Verification items for the finished model (mm, model axes). A direction names the side the tool comes from. Round coordinates to 2 decimals unless told otherwise and drop trailing zeros. Write each loop counter-clockwise with the first axis right and the second up, starting at its lowest first coordinate (ties: lowest second). Pieces come first, ordered by that corner, then holes. Notation, with made-up numbers: (6.5, 45.25) -> (65.5, 45.25) arc R21 cw to (65.5, 68.25) -> close; hole circle Ø1 at (41, 22.25). An arc over 180 degrees is marked (long way). Answer as a JSON object with one key per item and string values. Group by question number.
(1) Gauge pin test, flat ends, axial feed: pin 1 Ø16 at (x, y) = (-17, 7.5) entering from -Z; pin 2 Ø3 at (x, y) = (2.5, 34) entering from +Z; pin 3 Ø10 at (y, z) = (13, 18) entering from -X; pin 4 Ø3 at (x, z) = (4, 74) entering from -Y. Record the tip position at first contact, or that the pin passes through.
(2) Draft check along Z on faces 4 (the face through (-47, 10, -54)), 5 (the face through (-1, 80, -100)), 6 (the face through (-88.594, 80.14, 87.972)). Enter one of: released by +Z, released by -Z, zero draft, split by the parting line, or undercut.
(3) Sectioned sample at B-B on y = 77. Record the cut outline in (x, z), and give its area (3 significant figures).
(4) Scan lines: L1, parallel to X at y = 10.75, z = 50; L2, parallel to Y at x = 55, z = 47.5; L3, parallel to Y at x = -11, z = -85. Record each from-to range of solid material in increasing order. Write a range as from..to.
(5) Sectioned sample at A-A on x = 0. Record the cut outline in (y, z).
(6) Set-up check for faces 1 (the face through (-1, 20, -51)), 2 (the face through (-1, 10, -75)), 3 (the face through (68.986, 10.14, -69.297)): record each of +Z, -Z, +X, -X, +Y, -Y from which the full face is reachable in a straight line by a thin tool's end or side.
(7) Sectioned sample at D-D on z = 0. Record the cut outline in (x, y), and give its area (3 significant figures).
(8) Sectioned sample at C-C on z = -70. Record the cut outline in (x, y), and give its area (3 significant figures).
```python
from build123d import *

# Parameters (mm, degrees)
SKETCH_1_W      = 150
SKETCH_1_H      = 150
SKETCH_1_R      = 5
EXTRUDE_1_DEPTH = 20
FILLET_1_R      = 20
SKETCH_2_R      = 50
EXTRUDE_2_DEPTH = 50
SKETCH_3_W      = 200
SKETCH_3_H      = 200
EXTRUDE_3_DEPTH = 20
FILLET_2_R      = 40


with BuildPart() as part:
    # Эскиз1 → Бобышка-Вытянуть1 (new body)
    with BuildSketch(Plane(origin=(0, 0, 0), x_dir=(1, 0, 0), z_dir=(0, 1, 0))):
        Rectangle(SKETCH_1_W, SKETCH_1_H)
        with Locations(Location((-50, 50, 0), (0, 0, 270))):
            Circle(SKETCH_1_R, mode=Mode.SUBTRACT)
        with Locations(Location((50, 50, 0), (0, 0, 270))):
            Circle(SKETCH_1_R, mode=Mode.SUBTRACT)
        with Locations(Location((50, -50, 0), (0, 0, 270))):
            Circle(SKETCH_1_R, mode=Mode.SUBTRACT)
        with Locations(Location((-50, -50, 0), (0, 0, 270))):
            Circle(SKETCH_1_R, mode=Mode.SUBTRACT)
    extrude(amount=EXTRUDE_1_DEPTH)

    # Скругление1
    fillet_1_edges = [part.edges().sort_by_distance(p)[0] for p in [
        (-75, 10, 75),
        (-75, 10, -75),
        (75, 10, -75),
        (75, 10, 75),
    ]]
    fillet(fillet_1_edges, radius=FILLET_1_R)

    # Эскиз2 → Бобышка-Вытянуть2 (add)
    with BuildSketch(Plane(origin=(0, 20, 0), x_dir=(1, 0, 0), z_dir=(0, 1, 0))):
        with Locations(Location((0, 0, 0), (0, 0, 270))):
            Circle(SKETCH_2_R)
    extrude(amount=EXTRUDE_2_DEPTH)

    # Эскиз3 → Бобышка-Вытянуть3 (add)
    with BuildSketch(Plane(origin=(0, 70, 0), x_dir=(1, 0, 0), z_dir=(0, 1, 0))):
        Rectangle(SKETCH_3_W, SKETCH_3_H)
    extrude(amount=EXTRUDE_3_DEPTH)

    # Скругление2
    fillet_2_edges = [part.edges().sort_by_distance(p)[0] for p in [
        (100, 80, 100),
        (100, 80, -100),
        (-100, 80, -100),
        (-100, 80, 100),
    ]]
    fillet(fillet_2_edges, radius=FILLET_2_R)


solid = part.part
```
Computed values:
{
 "1": {"pin 1": "z = -75", "pin 2": "z = 49.99", "pin 3": "x = -75", "pin 4": "y = 0"},
 "2": {"face 4": "undercut", "face 5": "released by -Z", "face 6": "released by +Z"},
 "3": {"outline": "(-100, -60) arc R40 ccw to (-60, -100) -> (60, -100) arc R40 ccw to (100, -60) -> (100, 60) arc R40 ccw to (60, 100) -> (-60, 100) arc R40 ccw to (-100, 60) -> close", "area": "38,600 mm2"},
 "4": {"L1": "-75..-55, -45..45, 55..75", "L2": "0..20, 70..90", "L3": "70..90"},
 "5": {"outline": "(0, -75) -> (20, -75) -> (20, -50) -> (70, -50) -> (70, -100) -> (90, -100) -> (90, 100) -> (70, 100) -> (70, 50) -> (20, 50) -> (20, 75) -> (0, 75) -> close"},
 "6": {"face 1": "none", "face 2": "-Z, +X, -X, -Y", "face 3": "-Z, +X, -Y"},
 "7": {"outline": "(-100, 70) -> (-50, 70) -> (-50, 20) -> (-75, 20) -> (-75, 0) -> (75, 0) -> (75, 20) -> (50, 20) -> (50, 70) -> (100, 70) -> (100, 90) -> (-100, 90) -> close", "area": "12,000 mm2"},
 "8": {"outline": "(-98.73, 70) -> (98.73, 70) -> (98.73, 90) -> (-98.73, 90) -> close; (-68.23, 0) -> (68.23, 0) -> (68.23, 20) -> (-68.23, 20) -> close", "area": "6,680 mm2"}
}
